Autodesk Inventor part; units mm, degrees
ref_plane "YZ Plane" through (0, 0, 0) normal (1, 0, 0) x (0, 1, 0)
ref_plane "XZ Plane" through (0, 0, 0) normal (0, 1, 0) x (-1, 0, 0)
ref_plane "XY Plane" through (0, 0, 0) normal (0, 0, 1) x (1, 0, 0)
sketch "Sketch1" plane through (0, 0, 0) normal (0, 0, 1) x (1, 0, 0)
  line L0 (0, 0) -> (0, 70)
  line L1 (0, 70) -> (20, 70)
  line L2 (0, 0) -> (70, 0)
  line L3 (70, 0) -> (70, 20)
  arc A0 (20, 70) -> (70, 20) centre (111.1438, 111.1438) ccw
  arc A1 (23.5919, 44.5505) -> (44.5505, 23.5919) centre (111.1438, 111.1438) ccw
  line L4 (20, 43.3398) -> (20, 20)
  line L5 (20, 20) -> (43.3398, 20)
  arc A2 (23.5919, 44.5505) -> (20, 43.3398) centre (22, 43.3398) ccw
  arc A3 (43.3398, 20) -> (44.5505, 23.5919) centre (43.3398, 22) ccw
  line L6 (10, 62) -> (10, 30) construction
  line L7 (62, 10) -> (30, 10) construction
  circle A4 centre (10, 62) radius 2.5
  circle A5 centre (10, 30) radius 2.5
  circle A6 centre (30, 10) radius 2.5
  circle A7 centre (62, 10) radius 2.5
  point P0 (70, 10)
  point P1 (10, 70)
  dimension "d0" = 70
  dimension "d1" = 70
  dimension "d2" = 20
  dimension "d4" = 100
  dimension "d5" = 10
  dimension "d6" = 2
  dimension "d7" = 32
  dimension "d8" = 32
  dimension "d9" = 8
  dimension "d10" = 8
  dimension "d11" = 5
  dimension "d12" = 5
  dimension "d13" = 5
  dimension "d14" = 5
extrude "Extrusion1" add sketch "Sketch1" along normal mid plane 3.175
equation "\"d10\" = d9"
properties part number "Corner Bracket" material "Aluminum 6061"
Work out the finished part from the listing and answer in its coordinate system (mm). A direction names the side the tool comes from. Round coordinates to 2 decimals unless told otherwise and drop trailing zeros. Write each loop counter-clockwise with the first axis right and the second up, starting at its lowest first coordinate (ties: lowest second). Pieces come first, ordered by that corner, then holes. Notation, with made-up numbers: (46, -21) -> (85, -21) arc R11 cw to (85, -5) -> close; hole circle Ø4 at (66, -8). An arc over 180 degrees is marked (long way). Write each question's results on one line, items separated by ' | '.
Item 1: A cutting plane is placed at C-C, the plane x = 30. Determine the outline of the cut face in (y, z), plus the area to 3 significant figures.
Result set:
outline: (0, -1.59) -> (7.5, -1.59) -> (7.5, 1.59) -> (0, 1.59) -> close; (12.5, -1.59) -> (20, -1.59) -> (20, 1.59) -> (12.5, 1.59) -> close; (36.88, -1.59) -> (52.7, -1.59) -> (52.7, 1.59) -> (36.88, 1.59) -> close | area: 97.9 mm^2
Item 2: Find the intervals of material crossed by line 1 along Y through (x, z) = (10, -0.1); line 2 along Y through (x, z) = (30, -0.65); line 3 along X through (y, z) = (12, -0.45), in increasing order. Write a range as [from, to].
Result set:
line 1: [0, 27.5], [32.5, 59.5], [64.5, 70] | line 2: [0, 7.5], [12.5, 20], [36.88, 52.7] | line 3: [0, 28.5], [31.5, 60.5], [63.5, 70]
Item 3: A cutting plane is placed at A-A, the plane y = 10. Determine the outline of the cut face in (x, z).
Result set:
outline: (0, -1.59) -> (27.5, -1.59) -> (27.5, 1.59) -> (0, 1.59) -> close; (32.5, -1.59) -> (59.5, -1.59) -> (59.5, 1.59) -> (32.5, 1.59) -> close; (64.5, -1.59) -> (70, -1.59) -> (70, 1.59) -> (64.5, 1.59) -> close
Item 4: A cutting plane is placed at B-B, the plane z = 0.5. Determine the outline of the cut face in (x, y).
Result set:
outline: (0, 0) -> (70, 0) -> (70, 20) arc R100 cw to (20, 70) -> (0, 70) -> close; hole circle Ø5 at (10, 30); hole circle Ø5 at (10, 62); hole (20, 20) -> (43.34, 20) arc R2 ccw to (44.55, 23.59) arc R110 cw to (23.59, 44.55) arc R2 ccw to (20, 43.34) -> close; hole circle Ø5 at (30, 10); hole circle Ø5 at (62, 10)
Item 5: The mould has two halves that part along Y. Classify faces 1 (the face through (19, 28, -1.588)), 2 (the face through (10, 70, 0)), 3 (the face through (21.328, 45.224, -0.022)), 4 (the face through (45.246, 21.394, -0.022)): +Y half, -Y half, draft (parallel to the pull), parting line (faces both ways), or undercut.
Result set:
face 1: draft | face 2: +Y half | face 3: undercut | face 4: undercut
Item 6: Which of the six approach directions +Z, -Z, +X, -X, +Y, -Y give full straight-line access (tool end or side, diameter ignored) to faces 5 (the face through (32, 20, 0)), 6 (the face through (70, 10, 0))?
Result set:
face 5: +Z, -Z | face 6: +Z, -Z, +X, +Y, -Y
Item 7: A cutting plane is placed at D-D, the plane y = 62. Determine the outline of the cut face in (x, z), plus the area to 3 significant figures.
Result set:
outline: (0, -1.59) -> (7.5, -1.59) -> (7.5, 1.59) -> (0, 1.59) -> close; (12.5, -1.59) -> (24.05, -1.59) -> (24.05, 1.59) -> (12.5, 1.59) -> close | area: 60.5 mm^2
